The model under review builds one solid part; all positions refer to its coordinate system, in mm. Round coordinates to 2 decimals unless told otherwise and drop trailing zeros. Write each loop counter-clockwise with the first axis right and the second up, starting at its lowest first coordinate (ties: lowest second). Pieces come first, ordered by that corner, then holes. Notation, with made-up numbers: (-28.5, 44) - (3.5, 44) arc R21 cw to (3.5, 77) - close; hole circle Ø4 at (-1, 50.5). An arc over 180 degrees is marked (long way). Write each question's results on one line, items separated by ' | '.
```python
from build123d import *

# Parameters (mm, degrees)
SKETCH1_W           = 346.7
SKETCH1_H           = 357.50000001
BOSS_EXTRUDE1_DEPTH = 18
SKETCH2_W           = 346.7
SKETCH2_H           = 18
CUT_EXTRUDE1_DEPTH  = 6.35
FILLET1_R           = 9.525


with BuildPart() as part:
    # Sketch1 → Boss-Extrude1 (new body)
    with BuildSketch(Plane(origin=(0, 0, 0), x_dir=(1, 0, 0), z_dir=(0, 1, 0))):
        with Locations((173.35, -178.750000005)):
            Rectangle(SKETCH1_W, SKETCH1_H)
    extrude(amount=BOSS_EXTRUDE1_DEPTH)

    # Sketch2 → Cut-Extrude1 (cut)
    with BuildSketch(Plane(origin=(0, 18, 0), x_dir=(1, 0, 0), z_dir=(0, 1, 0))):
        with Locations((173.35, -310.40000001)):
            Rectangle(SKETCH2_W, SKETCH2_H)
    extrude(amount=-CUT_EXTRUDE1_DEPTH, mode=Mode.SUBTRACT)

    # Fillet1
    fillet1_edges = [part.edges().sort_by_distance(p)[0] for p in [
        (173.35, 0, 357.50000001),
    ]]
    fillet(fillet1_edges, radius=FILLET1_R)


solid = part.part
```
Q1. We need section C-C (z = 311.5). State the section outline as (x, y) points, plus the area to 3 significant figures.
Evaluation:
outline: (0, 0) - (346.7, 0) - (346.7, 11.65) - (0, 11.65) - close | area: 4,040 mm^2
Q2. The part is to be moulded in two halves that separate along Z. For faces 1 (the flat face through (171, 11.65, 310)), 2 (the flat face through (171, 14, 357.5)), 3 (the flat face through (171, 9, 0)), 4 (the flat face through (171, 18, 149)), say which applies: released by +Z, released by -Z, zero draft, split by the parting line, or undercut.
Evaluation:
face 1: undercut | face 2: released by +Z | face 3: released by -Z | face 4: zero draft
Q3. We need section A-A (y = 15). State the section outline as (x, z) points, plus the area to 3 significant figures.
Evaluation:
outline: (0, 0) - (346.7, 0) - (346.7, 301.4) - (0, 301.4) - close; (0, 319.4) - (346.7, 319.4) - (346.7, 357.5) - (0, 357.5) - close | area: 118,000 mm^2
Q4. Insertion check: P1, Ø8, axis at x = 45.5, y = 5, coming from the +Z side; P2, Ø1, axis at x = 103.5, y = 7, coming from the +Z side; P3, Ø4, axis at x = 296.5, y = 7, coming from the -Z side; P4, Ø3, axis at x = 42.5, y = 5.5, coming from the +Z side. Each pin has a flat end and moves straight along its axis. Give the tip position at first contact, or say it passes through.
Evaluation:
P1: stops at z = 357.49 | P2: stops at z = 357.28 | P3: stops at z = 0 | P4: stops at z = 357.16
Q5. We need section B-B (x = 53.5). State the section outline as (y, z) points (3 decimals).
Evaluation:
outline: (0, 0) - (18, 0) - (18, 301.4) - (11.65, 301.4) - (11.65, 319.4) - (18, 319.4) - (18, 357.5) - (9.525, 357.5) arc R9.525 ccw to (0, 347.975) - close
Q6. For probe 1 along Z at (x, y) = (302, 15.5); probe 2 along Z at (x, y) = (52, 9.25); probe 3 along Z at (x, y) = (183.5, 8.5), list the stretches that pass through material, from the lowest coordinate up.
Evaluation:
probe 1: z = 0 to 301.4, 319.4 to 357.5 | probe 2: z = 0 to 357.5 | probe 3: z = 0 to 357.44
